Autodesk Fusion 360 part; units mm, degrees
sketch "Sketch1" plane through (0, 0, 0) normal (0, 0, 1) x (1, 0, 0)
  line L0 (0, 0) -> (120, 0)
  line L1 (120, 0) -> (120, 40)
  line L2 (120, 40) -> (0, 40)
  arc A0 (0, 40) -> (0, 0) centre (0, 20) ccw
  line L3 (120, 40) -> (70, 40)
  line L4 (70, 40) -> (70, 30)
  line L5 (70, 30) -> (120, 30)
  line L6 (120, 30) -> (120, 40)
  line L7 (120, 0) -> (70, 0)
  line L8 (70, 0) -> (70, 10)
  line L9 (70, 10) -> (120, 10)
  line L10 (120, 10) -> (120, 0)
  line L11 (0, 30) -> (40, 30)
  line L12 (0, 10) -> (40, 10)
  arc A1 (0, 30) -> (0, 10) centre (0, 20) ccw
  arc A2 (40, 10) -> (40, 30) centre (40, 20) ccw
  dimension "d1" = 120
  dimension "d2" = 40
  dimension "d3" = 50
  dimension "d4" = 10
  dimension "d5" = 50
  dimension "d6" = 10
  dimension "d7" = 20
  dimension "d8" = 40
  dimension "d9" = 20
extrude "Extrude1" add sketch "Sketch1" along normal blind 10 contours L0 L1 L2 A0 L4 L5 L8 L9
extrude "Extrude2" add sketch "Sketch1" along normal blind 40 contours L0 L1 L7 L8 L9 L10 | L1 L2 L3 L4 L5 L6
sketch "Sketch2" plane through (0, 0, 0) normal (0, -1, 0) x (1, 0, 0)
  line L0 (0, 0) -> (120, 0)
  line L1 (120, 0) -> (120, 40)
  line L2 (120, 40) -> (70, 40)
  line L3 (70, 40) -> (70, 10)
  line L4 (70, 10) -> (0, 10)
  line L5 (0, 10) -> (0, 0)
  circle A0 centre (95, 40) radius 15
  arc A1 (120, 40) -> (70, 40) centre (95, 40) ccw
  dimension "d14" = 30
  dimension "d15" = 50
extrude "Extrude3" add sketch "Sketch2" against normal blind 10 contours L2 A0 A1
extrude "Extrude4" cut sketch "Sketch2" against normal blind 10 contours L2 A0 picked at (96.1126, 35.1254)
sketch "Sketch3" plane through (0, 40, 0) normal (0, 1, 0) x (-1, 0, 0)
  line L0 (-120, 0) -> (0, 0)
  line L1 (0, 0) -> (0, 10)
  line L2 (0, 10) -> (-70, 10)
  line L3 (-70, 10) -> (-70, 40)
  line L4 (-70, 40) -> (-120, 40)
  line L5 (-120, 40) -> (-120, 0)
  circle A0 centre (-95, 40) radius 15
  arc A1 (-70, 40) -> (-120, 40) centre (-95, 40) ccw
  dimension "d20" = 30
  dimension "d21" = 50
extrude "Extrude5" cut sketch "Sketch3" against normal blind 10 contours L4 A0 picked at (-93.8874, 35.1254)
extrude "Extrude6" add sketch "Sketch3" against normal blind 10 contours L4 A0 A1
Build history of the part. All positions in model axes, mm. A direction names the side the tool comes from. Round coordinates to 2 decimals unless told otherwise and drop trailing zeros. Write each loop counter-clockwise with the first axis right and the second up, starting at its lowest first coordinate (ties: lowest second). Pieces come first, ordered by that corner, then holes. Notation, with made-up numbers: (-6, -12) - (10, -12) arc R14 ccw to (10, 10) - close; hole circle Ø3 at (-33.75, -34). An arc over 180 degrees is marked (long way). Use CSV: the item, a comma, the result in double quotes.
(1) Mould opens along X. For faces 1 (the flat face through (70, 35, 25)), 2 (the flat face through (20, 30, 5)), 3 (the flat face through (120, 20, 6)), 4 (the cylindrical face through (86.94, 35.07, 52.65)) say: pulls with the +X half, pulls with the -X half, needs draft (parallel to the pull), parting line crosses it, or undercut.
Response:
face 1,"pulls with the -X half"
face 2,"undercut"
face 3,"pulls with the +X half"
face 4,"undercut"
(2) Band-saw the part on C-C (x = 5). Write the cut outline in (y, z).
Response:
outline,"(0, 0) - (10, 0) - (10, 10) - (0, 10) - close; (30, 0) - (40, 0) - (40, 10) - (30, 10) - close"
(3) Band-saw the part on B-B (z = 12). Write the cut outline in (x, y), plus the area to 3 significant figures.
Response:
outline,"(70, 0) - (120, 0) - (120, 10) - (70, 10) - close; (70, 30) - (120, 30) - (120, 40) - (70, 40) - close"
area,"1,000 mm²"
(4) Band-saw the part on D-D (z = 50). Write the cut outline in (x, y), plus the area to 3 significant figures.
Response:
outline,"(72.09, 0) - (83.82, 0) - (83.82, 10) - (72.09, 10) - close; (72.09, 30) - (83.82, 30) - (83.82, 40) - (72.09, 40) - close; (106.18, 0) - (117.91, 0) - (117.91, 10) - (106.18, 10) - close; (106.18, 30) - (117.91, 30) - (117.91, 40) - (106.18, 40) - close"
area,"469 mm²"
(5) Band-saw the part on A-A (x = 95). Write the cut outline in (y, z).
Response:
outline,"(0, 0) - (40, 0) - (40, 25) - (30, 25) - (30, 10) - (10, 10) - (10, 25) - (0, 25) - close; (0, 55) - (10, 55) - (10, 65) - (0, 65) - close; (30, 55) - (40, 55) - (40, 65) - (30, 65) - close"
(6) Pin check, flat tips, straight feed: P1, Ø5, axis at y = 8.5, z = 23, coming from the -X side; P2, Ø1, axis at x = 47.5, y = 33.5, coming from the +Z side; P3, Ø1.5, axis at x = 105.5, y = 8.5, coming from the +Z side; P4, Ø24, axis at x = 95, z = 40, coming from the -Y side. Stop position of each tip, or through.
Response:
P1,"x = 70"
P2,"z = 10"
P3,"z = 63.02"
P4,"through"
(7) 3-axis set-ups, long thin cutter, end or side, ignore diameter. For faces 5 (the cylindrical face through (50, 20, 5)), 6 (the cylindrical face through (103.06, 4.93, 52.65)), 7 (the flat face through (70, 5, 25)), 8 (the flat face through (89.8, 30, 25.7)): which of +Z, -Z, +X, -X, +Y, -Y reach the whole face in a straight line?
Response:
face 5,"+Z, -Z"
face 6,"+Y, -Y"
face 7,"+Z, -X, +Y, -Y"
face 8,"+Z, +X, -X"
(8) Wall check: line 1 (Z direction, x = 95, y = 7); line 2 (X direction, y = 35.5, z = 40); line 3 (Y direction, x = 71, z = 15). Give the ranges that are in metal, low to high.
Response:
line 1,"0 to 25, 55 to 65"
line 2,"70 to 80, 110 to 120"
line 3,"0 to 10, 30 to 40"
